from build123d import *

# Parameters (mm, degrees)
SKETCH_1_R          = 8
EXTRUDE_1_DEPTH     = 4
SKETCH_2_R          = 6
EXTRUDE_2_DEPTH     = 18
SKETCH_3_R          = 4
CUT_EXTRUDE_1_DEPTH = 23
CHAMFER_1_SIZE      = 1


with BuildPart() as part:
    # 스케치1 → 보스-돌출1 (new body)
    with BuildSketch(Plane.XY):
        Circle(SKETCH_1_R)
    extrude(amount=EXTRUDE_1_DEPTH)

    # 스케치2 → 보스-돌출2 (add)
    with BuildSketch(Plane(origin=(0, 0, 0), x_dir=(-1, 0, 0), z_dir=(0, 0, -1))):
        Circle(SKETCH_2_R)
    extrude(amount=EXTRUDE_2_DEPTH)

    # 스케치3 → 컷-돌출1 (cut, through all)
    with BuildSketch(Plane(origin=(0, 0, -18), x_dir=(-1, 0, 0), z_dir=(0, 0, -1))):
        Circle(SKETCH_3_R)
    extrude(amount=-CUT_EXTRUDE_1_DEPTH, mode=Mode.SUBTRACT)

    # 모따기1
    chamfer_1_edges = [part.edges().sort_by_distance(p)[0] for p in [
        (-8, 0, 4),
        (6, 0, -18),
    ]]
    chamfer(chamfer_1_edges, length=CHAMFER_1_SIZE)


solid = part.part
Can you work these out from the model? Positions are in its coordinate system, mm. A direction names the side the tool comes from. Round coordinates to 2 decimals unless told otherwise and drop trailing zeros. Write each loop counter-clockwise with the first axis right and the second up, starting at its lowest first coordinate (ties: lowest second). Pieces come first, ordered by that corner, then holes. Notation, with made-up numbers: (37, -17) - (59, -17) arc R12 cw to (59, -1) - close; hole circle Ø9 at (52, 13.25). An arc over 180 degrees is marked (long way). Write each question's results on one line, items separated by ' | '. Start each with the question number.
1) We'd pull the mould along Y, two halves only. Please class faces 3 (the cylindrical face through (0.867, -3.905, -7.154)), 4 (the flat face through (-2, 6, 0)), 5 (the cylindrical face through (-1.73, -7.81, 1.48)): released by +Y, released by -Y, zero draft, split by the parting line, or undercut.
2) Suppose I cut it at A-A (x = 0). List the corners of the cut face in (y, z) for me, and give its area (3 significant figures).
3) Please list where these lines run through material, in increasing order: line 1 (Y direction, x = 0, z = -7); line 2 (X direction, y = -2.75, z = -9); line 3 (Y direction, x = 1.25, z = -0.5).
4) For pin 1 Ø4 at (y, z) = (-5.5, 1.5) entering from -X; pin 2 Ø6 at (x, z) = (-4, -8.5) entering from +Y; pin 3 Ø8 at (x, z) = (0, -12) entering from -Y, each with a flat end and sliding along its axis, tell me the tip position at first contact or that it passes through.
5) Suppose I cut it at C-C (z = -3.5). List the corners of the cut face in (x, y) for me.
6) Which directions (+Z, -Z, +X, -X, +Y, -Y) give clear straight access to the entire face, cutting with the end or side of a thin tool? Please do faces 1 (the cylindrical face through (6, 0, -8)), 2 (the flat face through (3, -3, 4)).
Here are the results:
1) face 3: undercut | face 4: zero draft | face 5: split by the parting line
2) outline: (-8, 0) - (-6, 0) - (-6, -17) - (-5, -18) - (-4, -18) - (-4, 4) - (-7, 4) - (-8, 3) - close; (4, -18) - (5, -18) - (6, -17) - (6, 0) - (8, 0) - (8, 3) - (7, 4) - (4, 4) - close | area: 102 mm2
3) line 1: y = -6 to -4, 4 to 6 | line 2: x = -5.33 to -2.9, 2.9 to 5.33 | line 3: y = -5.87 to -3.8, 3.8 to 5.87
4) pin 1: stops at x = -7.19 | pin 2: stops at y = 5.92 | pin 3: stops at y = -6
5) outline: circle Ø12 at (0, 0); hole circle Ø8 at (0, 0)
6) face 1: -Z | face 2: +Z, +X, -X, +Y, -Y
